Autodesk Inventor part; units mm, degrees
ref_plane "Начальная плоскость" through (0, 0, 50) normal (0, 0, 1) x (1, 0, 0)
ref_plane "Конечная плоскость" through (0, 0, 1450) normal (0, 0, 1) x (1, 0, 0)
ref_plane "РабПлоскость4" through (25, -1000, 50) normal (0, 0, -1) x (-1, 0, 0)
ref_plane "Начальная плоскость" through (0, 0, 50) normal (0, 0, 1) x (1, 0, 0)
ref_plane "Конечная плоскость" through (0, 0, 1450) normal (0, 0, 1) x (1, 0, 0)
sketch "Эскиз" plane through (0, 0, 0) normal (0, 0, 1) x (1, 0, 0)
  circle A0 centre (0, 0) radius 16.15
  circle A1 centre (0, 0) radius 24.15
  dimension "d0" = 48.3
  dimension "d1" = 8
extrude "Тело" add sketch "Эскиз" along normal up to surface (1400 mm away) from surface at 50
sketch "Sketch3" plane through (0, 0, 0) normal (0, 0, 1) x (1, 0, 0)
  line L0 (0, 0) -> (10, 0)
ref_plane "Work Plane3" through (0, 0, 0) normal (0, -1, 0) x (1, 0, 0)
sketch "Sketch4" plane through (0, 0, 0) normal (0, -1, 0) x (1, 0, 0)
  line L0 (-2, 50) -> (12, 50)
  line L1 (-2, 1450) -> (12, 1450)
  dimension "d7" = 1400
ref_plane "РабПлоскость4" through (25, -1000, 50) normal (0, 0, -1) x (-1, 0, 0)
split "Разделение1" plane through (25, -1000, 50) removes the side toward (0, 0, -1)
ref_plane "РабПлоскость5" through (-25, -1000, 1450) normal (0, 0, 1) x (1, 0, 0)
split "Разделение2" plane through (-25, -1000, 1450) removes the side toward (0, 0, 1)
equation "\"d0\" = G_H"
equation "\"d1\" = G_T"
equation "\"d2\" = G_L"
equation "\"G_H\" = 48.3"
equation "\"G_T\" = 8"
equation "\"G_L\" = d7"
properties part number "DIN2448 - 48,3 x 8 - 1400" material "Сталь, мягкая"
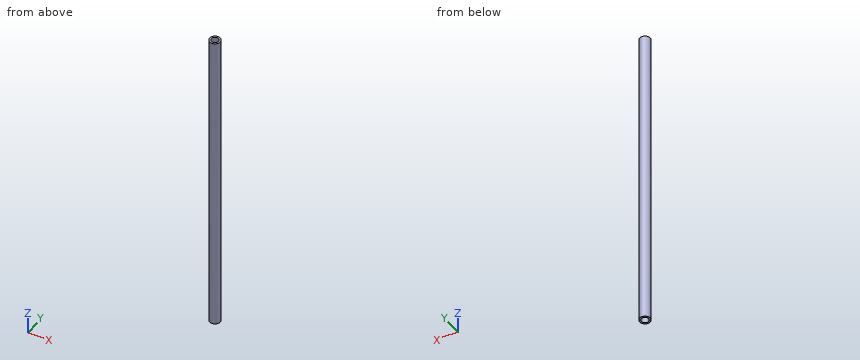
Part model, mm, in its own coordinate system. Round coordinates to 2 decimals unless told otherwise and drop trailing zeros. Write each loop counter-clockwise with the first axis right and the second up, starting at its lowest first coordinate (ties: lowest second). Pieces come first, ordered by that corner, then holes. Notation, with made-up numbers: (39.5, -27.75) -> (43.5, -27.75) arc R21 cw to (43.5, -9.75) -> close; hole circle Ø1 at (84, -37). An arc over 180 degrees is marked (long way). Return JSON: item names as keys, results as strings. Group by question number.
Q1. Saw through at C-C on z = 382. Write the cut outline in (x, y), plus the area to 3 significant figures.
Q2. Saw through at A-A on x = 0. Write the cut outline in (y, z), plus the area to 3 significant figures.
Q3. Pin check, flat tips, straight feed: pin 1 (2 mm diameter, centred on y = -12, z = 1156, fed in from -X); pin 2 (1.5 mm diameter, centred on x = 10, z = 1054.5, fed in from +Y); pin 3 (12 mm diameter, centred on x = 4.5, y = -3.5, fed in from -Z); pin 4 (2 mm diameter, centred on x = 14, z = 963.5, fed in from -Y). Stop position of each tip, or through.
Q4. Probe L1, parallel to Y at x = 0, z = 1104; L2, parallel to X at y = 2.5, z = 639; L3, parallel to X at y = 6, z = 352. List the from-to ranges inside material, lowest first. Write a range as [from, to].
Answer:
{
 "1": {"outline": "circle Ø48.3 at (0, 0); hole circle Ø32.3 at (0, 0)", "area": "1,010 mm2"},
 "2": {"outline": "(-24.15, 50) -> (-16.15, 50) -> (-16.15, 1450) -> (-24.15, 1450) -> close; (16.15, 50) -> (24.15, 50) -> (24.15, 1450) -> (16.15, 1450) -> close", "area": "22,400 mm2"},
 "3": {"pin 1": "x = -21.5", "pin 2": "y = 22.31", "pin 3": "through", "pin 4": "y = -20.35"},
 "4": {"L1": "[-24.15, -16.15], [16.15, 24.15]", "L2": "[-24.02, -15.96], [15.96, 24.02]", "L3": "[-23.39, -14.99], [14.99, 23.39]"}
}
